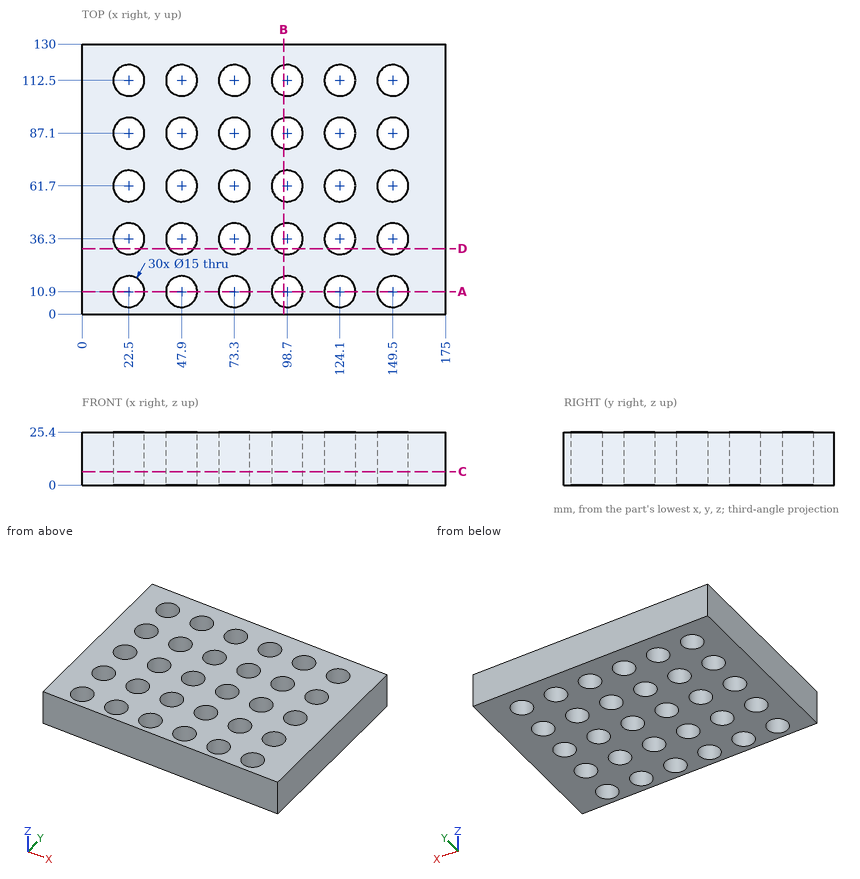
Job drawing, mm, ordinate dimensions from the low corner. One solid piece. Coordinates: 2 decimals unless noted, no trailing zeros. Order: outer loops, then holes, each group sorted by start corner. A loop starts at its lowest first (then second) coordinate and runs counter-clockwise, first axis right, second up. Notation, with made-up numbers: (53.25, 72.5) -> (101.25, 72.5) arc R16 cw to (101.25, 94.5) -> close; hole circle Ø8 at (-38.5, -15.75). An arc over 180 degrees is marked (long way). Answer in a Markdown table with one row per item. Add a question column.
Q1. Band-saw the part on A-A, the plane y = 10.9. List the corners of the cut face in (x, z).
Q2. Wall check: line 1 along Y through (x, z) = (22.5, 13.25); line 2 along Y through (x, z) = (154.5, 8.25). Give the ranges that are in metal, low to high. Write a range as [from, to].
Q3. Band-saw the part on B-B, the plane x = 97. List the corners of the cut face in (y, z), then the cut area to 3 significant figures.
Q4. Band-saw the part on C-C, the plane z = 6.5. Give the number of separate pieces and of enclosed holes in the cut face, then the cut area to 3 significant figures.
Q5. Band-saw the part on D-D, the plane y = 31.5. List the corners of the cut face in (x, z), then the cut area to 3 significant figures.
Q6. Drop a flat-ended pin along its axis: pin 1 (19.5 mm diameter, centred on x = 22.5, y = 112.5, fed in from +Z). Give the stop position or say it passes through.
Answers follow:
| question | item | result |
|---|---|---|
| 1 | outline | (0, 0) -> (15, 0) -> (15, 25.4) -> (0, 25.4) -> close; (30, 0) -> (40.4, 0) -> (40.4, 25.4) -> (30, 25.4) -> close; (55.4, 0) -> (65.8, 0) -> (65.8, 25.4) -> (55.4, 25.4) -> close; (80.8, 0) -> (91.2, 0) -> (91.2, 25.4) -> (80.8, 25.4) -> close; (106.2, 0) -> (116.6, 0) -> (116.6, 25.4) -> (106.2, 25.4) -> close; (131.6, 0) -> (142, 0) -> (142, 25.4) -> (131.6, 25.4) -> close; (157, 0) -> (175, 0) -> (175, 25.4) -> (157, 25.4) -> close |
| 2 | line 1 | [0, 3.4], [18.4, 28.8], [43.8, 54.2], [69.2, 79.6], [94.6, 105], [120, 130] |
| 2 | line 2 | [0, 5.31], [16.49, 30.71], [41.89, 56.11], [67.29, 81.51], [92.69, 106.91], [118.09, 130] |
| 3 | outline | (0, 0) -> (3.6, 0) -> (3.6, 25.4) -> (0, 25.4) -> close; (18.2, 0) -> (29, 0) -> (29, 25.4) -> (18.2, 25.4) -> close; (43.6, 0) -> (54.4, 0) -> (54.4, 25.4) -> (43.6, 25.4) -> close; (69, 0) -> (79.8, 0) -> (79.8, 25.4) -> (69, 25.4) -> close; (94.4, 0) -> (105.2, 0) -> (105.2, 25.4) -> (94.4, 25.4) -> close; (119.8, 0) -> (130, 0) -> (130, 25.4) -> (119.8, 25.4) -> close |
| 3 | area | 1,450 mm^2 |
| 4 | separate pieces | 1 |
| 4 | enclosed holes | 30 |
| 4 | area | 17,400 mm^2 |
| 5 | outline | (0, 0) -> (16.74, 0) -> (16.74, 25.4) -> (0, 25.4) -> close; (28.26, 0) -> (42.14, 0) -> (42.14, 25.4) -> (28.26, 25.4) -> close; (53.66, 0) -> (67.54, 0) -> (67.54, 25.4) -> (53.66, 25.4) -> close; (79.06, 0) -> (92.94, 0) -> (92.94, 25.4) -> (79.06, 25.4) -> close; (104.46, 0) -> (118.34, 0) -> (118.34, 25.4) -> (104.46, 25.4) -> close; (129.86, 0) -> (143.74, 0) -> (143.74, 25.4) -> (129.86, 25.4) -> close; (155.26, 0) -> (175, 0) -> (175, 25.4) -> (155.26, 25.4) -> close |
| 5 | area | 2,690 mm^2 |
| 6 | pin 1 | z = 25.4 |
